The listing builds one solid part. Answer for the finished solid, in the listing's coordinates (mm). Round coordinates to 2 decimals unless told otherwise and drop trailing zeros. Loops run counter-clockwise (first coordinate to the right, second up) from the corner with the lowest first, then second, coordinate; pieces in that order, holes last. Notation, with made-up numbers: (65.25, 29) - (90.25, 29) arc R19 cw to (90.25, 44) - close; hole circle Ø3 at (-14, 48). An arc over 180 degrees is marked (long way). One line per item, written item: value.
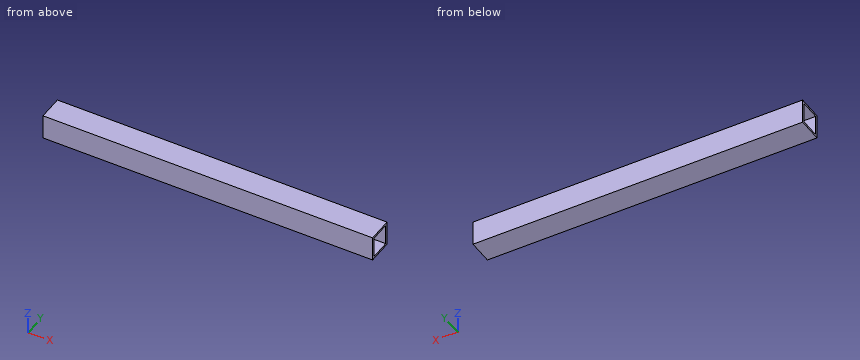
```python
from build123d import *

# Parameters (mm, degrees)
SKETCH_W       = 31.75
SKETCH_H       = 31.75
SKETCH_W_2     = 26.2128
SKETCH_H_2     = 26.2128
PAD_DEPTH      = 211.137
PAD_DEPTH_BACK = 211.137


with BuildPart() as part:
    # Sketch → Pad (new body, two sides)
    with BuildSketch(Plane.YZ) as pad_sk:
        Rectangle(SKETCH_W, SKETCH_H)
        Rectangle(SKETCH_W_2, SKETCH_H_2, mode=Mode.SUBTRACT)
    extrude(amount=PAD_DEPTH)
    extrude(pad_sk.sketch, amount=-PAD_DEPTH_BACK)


solid = part.part
```
1) A cutting plane is placed at C-C on x = 151. Give the vertices of the cut face in (y, z) (3 decimals).
Final values:
outline: (-15.875, -15.875) - (15.875, -15.875) - (15.875, 15.875) - (-15.875, 15.875) - close; hole (-13.106, -13.106) - (13.106, -13.106) - (13.106, 13.106) - (-13.106, 13.106) - close
2) Consider L1, parallel to Z at x = 158, y = 5.5 (3 decimals). Determine where the line is inside the solid, lowest interval first.
Final values:
L1: -15.875 to -13.106, 13.106 to 15.875
3) A cutting plane is placed at A-A on y = 6.5. Give the vertices of the cut face in (x, z) (3 decimals).
Final values:
outline: (-211.137, -15.875) - (211.137, -15.875) - (211.137, -13.106) - (-211.137, -13.106) - close; (-211.137, 13.106) - (211.137, 13.106) - (211.137, 15.875) - (-211.137, 15.875) - close
